from build123d import *

# Parameters (mm, degrees)
SKETCH1_W      = 95.25
SKETCH1_H      = 19.05
EXTRUDE1_DEPTH = 80.9625
CHAMFER1_SIZE  = 9.525
SKETCH6_W      = 161.925
SKETCH6_H      = 63.5
EXTRUDE2_DEPTH = 1.016
EXTRUDE5_DEPTH = 80.9625
EXTRUDE8_DEPTH = 20.05
CHAMFER8_SIZE  = 0.762
EXTRUDE9_DEPTH = 19.034
CHAMFER9_SIZE  = 3.048
CHAMFER6_SIZE  = 0.762


with BuildPart() as part:
    # Sketch1 → Extrude1 (new body, symmetric)
    with BuildSketch(Plane(origin=(0, 0, 0), x_dir=(0, 0, -1), z_dir=(1, 0, 0))):
        with Locations((0, 9.525)):
            Rectangle(SKETCH1_W, SKETCH1_H)
    extrude(amount=EXTRUDE1_DEPTH, both=True)

    # Chamfer1
    chamfer1_edges = [part.edges().sort_by_distance(p)[0] for p in [
        (80.9625, 9.525, 47.625),
        (-80.9625, 9.525, 47.625),
    ]]
    chamfer(chamfer1_edges, length=CHAMFER1_SIZE)

    # Sketch6 → Extrude2 (cut)
    with BuildSketch(Plane(origin=(0, 19.05, 0), x_dir=(1, 0, 0), z_dir=(0, 1, 0))):
        Rectangle(SKETCH6_W, SKETCH6_H)
    extrude(amount=-EXTRUDE2_DEPTH, mode=Mode.SUBTRACT)

    # Sketch10 → Extrude5 (add, symmetric)
    with BuildSketch(Plane(origin=(0, 0, 0), x_dir=(0, 0, -1), z_dir=(1, 0, 0))):
        with BuildLine():
            Line((47.117, 19.05), (47.117, 0))
            Line((47.117, 0), (49.657, 0))
            Line((49.657, 0), (49.657, 18.314590334))
            ThreePointArc((49.657, 18.314590334), (48.705491945, 18.860491945), (47.625, 19.05))
            Line((47.625, 19.05), (47.117, 19.05))
        make_face()
    extrude(amount=EXTRUDE5_DEPTH, both=True)

    # Sketch16 → Extrude8 (cut, through all)
    with BuildSketch(Plane.XZ):
        with BuildLine():
            Line((-54.9275, 24.765), (-54.9275, 19.685))
            ThreePointArc((-54.9275, 19.685), (-61.9125, 12.7), (-68.8975, 19.685))
            Line((-68.8975, 19.685), (-68.8975, 24.765))
            ThreePointArc((-68.8975, 24.765), (-61.9125, 31.75), (-54.9275, 24.765))
        make_face()
        with BuildLine():
            Line((-54.9275, -19.685), (-54.9275, -24.765))
            ThreePointArc((-54.9275, -24.765), (-61.9125, -31.75), (-68.8975, -24.765))
            Line((-68.8975, -24.765), (-68.8975, -19.685))
            ThreePointArc((-68.8975, -19.685), (-61.9125, -12.7), (-54.9275, -19.685))
        make_face()
        with BuildLine():
            Line((-13.6525, -19.685), (-13.6525, -24.765))
            ThreePointArc((-13.6525, -24.765), (-20.6375, -31.75), (-27.6225, -24.765))
            Line((-27.6225, -24.765), (-27.6225, -19.685))
            ThreePointArc((-27.6225, -19.685), (-20.6375, -12.7), (-13.6525, -19.685))
        make_face()
        with BuildLine():
            Line((27.6225, -19.685), (27.6225, -24.765))
            ThreePointArc((27.6225, -24.765), (20.6375, -31.75), (13.6525, -24.765))
            Line((13.6525, -24.765), (13.6525, -19.685))
            ThreePointArc((13.6525, -19.685), (20.6375, -12.7), (27.6225, -19.685))
        make_face()
        with BuildLine():
            Line((68.8975, -19.685), (68.8975, -24.765))
            ThreePointArc((68.8975, -24.765), (61.9125, -31.75), (54.9275, -24.765))
            Line((54.9275, -24.765), (54.9275, -19.685))
            ThreePointArc((54.9275, -19.685), (61.9125, -12.7), (68.8975, -19.685))
        make_face()
        with BuildLine():
            Line((68.8975, 24.765), (68.8975, 19.685))
            ThreePointArc((68.8975, 19.685), (61.9125, 12.7), (54.9275, 19.685))
            Line((54.9275, 19.685), (54.9275, 24.765))
            ThreePointArc((54.9275, 24.765), (61.9125, 31.75), (68.8975, 24.765))
        make_face()
        with BuildLine():
            Line((27.6225, 24.765), (27.6225, 19.685))
            ThreePointArc((27.6225, 19.685), (20.6375, 12.7), (13.6525, 19.685))
            Line((13.6525, 19.685), (13.6525, 24.765))
            ThreePointArc((13.6525, 24.765), (20.6375, 31.75), (27.6225, 24.765))
        make_face()
        with BuildLine():
            Line((-13.6525, 24.765), (-13.6525, 19.685))
            ThreePointArc((-13.6525, 19.685), (-20.6375, 12.7), (-27.6225, 19.685))
            Line((-27.6225, 19.685), (-27.6225, 24.765))
            ThreePointArc((-27.6225, 24.765), (-20.6375, 31.75), (-13.6525, 24.765))
        make_face()
    extrude(amount=-EXTRUDE8_DEPTH, mode=Mode.SUBTRACT)

    # Chamfer8
    chamfer8_edges = [part.edges().sort_by_distance(p)[0] for p in [
        (-20.6375, 0, -12.7),
        (-27.6225, 0, -22.225),
        (-20.6375, 0, -31.75),
        (-13.6525, 0, -22.225),
        (20.6375, 0, -12.7),
        (13.6525, 0, -22.225),
        (20.6375, 0, -31.75),
        (27.6225, 0, -22.225),
        (61.9125, 0, -12.7),
        (54.9275, 0, -22.225),
        (61.9125, 0, -31.75),
        (68.8975, 0, -22.225),
        (61.9125, 0, 31.75),
        (54.9275, 0, 22.225),
        (61.9125, 0, 12.7),
        (68.8975, 0, 22.225),
        (20.6375, 0, 31.75),
        (13.6525, 0, 22.225),
        (20.6375, 0, 12.7),
        (27.6225, 0, 22.225),
        (-20.6375, 0, 31.75),
        (-27.6225, 0, 22.225),
        (-20.6375, 0, 12.7),
        (-13.6525, 0, 22.225),
        (-61.9125, 0, 31.75),
        (-68.8975, 0, 22.225),
        (-61.9125, 0, 12.7),
        (-54.9275, 0, 22.225),
        (-61.9125, 0, -12.7),
        (-68.8975, 0, -22.225),
        (-61.9125, 0, -31.75),
        (-54.9275, 0, -22.225),
    ]]
    chamfer(chamfer8_edges, length=CHAMFER8_SIZE)

    # Sketch17 → 1/2 (0.5) Diameter Hole2 (revolve, cut)
    with BuildSketch(Plane(origin=(47.625, 18.034, 0), x_dir=(0, 0, 1), z_dir=(1, 0, 0))):
        Polygon((0, 0), (0, 18.034), (9.525, 18.034), (6.3754, 14.8844), (6.3754, 3.1496), (9.525, 0), align=None)
    revolve(axis=Axis((47.625, 24.384, 0), (0, -1, 0)), mode=Mode.SUBTRACT)

    # Sketch20 → Extrude9 (cut, through all)
    with BuildSketch(Plane(origin=(0, 18.034, 0), x_dir=(1, 0, 0), z_dir=(0, 1, 0))):
        with BuildLine():
            Line((-48.895, 6.3754), (-46.355, 6.3754))
            ThreePointArc((-46.355, 6.3754), (-39.9796, 0), (-46.355, -6.3754))
            Line((-46.355, -6.3754), (-48.895, -6.3754))
            ThreePointArc((-48.895, -6.3754), (-55.2704, 0), (-48.895, 6.3754))
        make_face()
    extrude(amount=-EXTRUDE9_DEPTH, mode=Mode.SUBTRACT)

    # Chamfer9
    chamfer9_edges = [part.edges().sort_by_distance(p)[0] for p in [
        (-55.2704, 0, 0),
        (-47.625, 0, -6.3754),
        (-39.9796, 0, 0),
        (-47.625, 0, 6.3754),
        (-55.2704, 18.034, 0),
        (-47.625, 18.034, 6.3754),
        (-39.9796, 18.034, 0),
        (-47.625, 18.034, -6.3754),
    ]]
    chamfer(chamfer9_edges, length=CHAMFER9_SIZE)

    # Chamfer6
    chamfer6_edges = [part.edges().sort_by_distance(p)[0] for p in [
        (80.9625, 19.05, -39.6875),
        (0, 0, 47.625),
        (0, 19.05, 47.625),
        (-80.9625, 0, -5.7785),
        (80.9625, 0, -5.7785),
        (76.2, 0, 42.8625),
        (-76.2, 0, 42.8625),
        (76.2, 19.05, 42.8625),
        (-76.2, 19.05, 42.8625),
        (-80.9625, 19.05, 34.925),
        (80.9625, 19.05, 34.925),
        (0, 19.05, 31.75),
        (0, 19.05, -31.75),
        (-80.9625, 19.05, -39.6875),
        (80.9625, 9.157295167, -49.657),
        (80.9625, 18.860491945, -48.705491945),
        (0, 0, -49.657),
        (-80.9625, 18.860491945, -48.705491945),
        (-80.9625, 9.157295167, -49.657),
    ]]
    chamfer(chamfer6_edges, length=CHAMFER6_SIZE)


solid = part.part
For this review, take the finished solid that the model builds, in its own axes (mm). A direction names the side the tool comes from. Round coordinates to 2 decimals unless told otherwise and drop trailing zeros. Loops run counter-clockwise (first coordinate to the right, second up) from the corner with the lowest first, then second, coordinate; pieces in that order, holes last. Notation, with made-up numbers: (-34.5, 78) - (-10.5, 78) arc R10 ccw to (-10.5, 84) - close; hole circle Ø9 at (6, 77). An arc over 180 degrees is marked (long way). Answer as CSV lines item,"result".
(1) Mouldability with a two-part tool opening along Z and no side actions: class faces 1 (the face through (-54.928, 9, -22)), 2 (the face through (-75.868, 0.386, 42.664)) as +Z half, -Z half, draft (parallel to the pull), parting line (faces both ways), or undercut.
Checked values:
face 1,"undercut"
face 2,"+Z half"
(2) Wall thickness on line 1 (X direction, y = 9.5, z = 0); line 2 (X direction, y = 2.25, z = 30.5); line 3 (Z direction, x = -15, y = 2) (3 decimals): over which ranges is each line inside the solid? List them lowest first.
Checked values:
line 1,"x = -80.96 to -55.27, -39.98 to 41.25, 54 to 80.96"
line 2,"x = -80.96 to -65.9, -57.93 to -24.62, -16.65 to 16.65, 24.62 to 57.93, 65.9 to 80.96"
line 3,"z = -49.657 to -28.889, -15.561 to 15.561, 28.889 to 47.625"
(3) Consider section A-A on z = 0. Give the boundary of the cut face in (x, y).
Checked values:
outline,"(-80.96, 0.76) - (-80.2, 0) - (-58.32, 0) - (-55.27, 3.05) - (-55.27, 14.99) - (-58.32, 18.03) - (-80.96, 18.03) - close; (-39.98, 3.05) - (-36.93, 0) - (38.1, 0) - (41.25, 3.15) - (41.25, 14.88) - (38.1, 18.03) - (-36.93, 18.03) - (-39.98, 14.99) - close; (54, 3.15) - (57.15, 0) - (80.2, 0) - (80.96, 0.76) - (80.96, 18.03) - (57.15, 18.03) - (54, 14.88) - close"
(4) Tool access review of faces 3 (the face through (-13.652, 9, -22)), 4 (the face through (-62.07, 0.64, -12.58)), 5 (the face through (53.456, 15.081, 3.033)): name each direction out of +Z, -Z, +X, -X, +Y, -Y from which nothing blocks a thin tool from reaching the whole face with its end or side.
Checked values:
face 3,"+Y, -Y"
face 4,"-Y"
face 5,"+Y"
(5) Insertion check: P1, Ø10, axis at x = 10, z = -2.5, coming from the +Y side; P2, Ø8, axis at x = 53, z = -0.5, coming from the +Y side. Each pin has a flat end and moves straight along its axis. Give the tip position at first contact, or say it passes through.
Checked values:
P1,"stops at y = 18.03"
P2,"stops at y = 17.91"
(6) Consider section B-B on y = 11. Give the number of separate pieces and of enclosed holes in the cut face, then the cut area to 3 significant figures.
Checked values:
separate pieces,"1"
enclosed holes,"10"
area,"13,600 mm2"
